For this review, use the dimensioned drawing (mm, ordinates from the lowest corner) and the shaded views. A direction names the side the tool comes from. Give positions to 0.01 mm unless a question says otherwise; leave off trailing zeros. Order: outer loops, then holes, each group sorted by start corner. A loop starts at its lowest first (then second) coordinate and runs counter-clockwise, first axis right, second up. Notation, with made-up numbers: (71, 89) - (117, 89) arc R30 ccw to (117, 121) - close; hole circle Ø9 at (38.25, 44.25). An arc over 180 degrees is marked (long way). Answer as CSV lines item,"result". Start each with the question number.
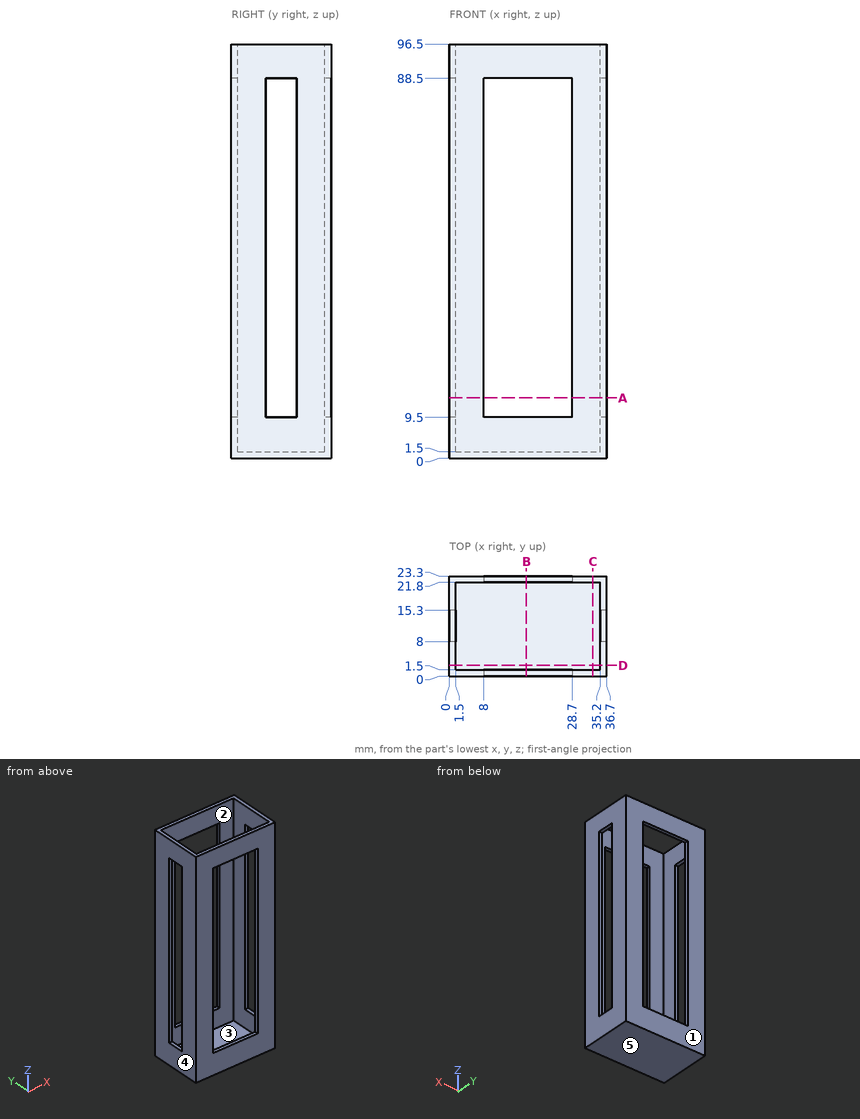
Item 1: Machinability: for the marked faces 1 and 2, which of the approach directions +Z, -Z, +X, -X, +Y, -Y give a long, thin tool a straight path to every point of the face, cutting with its end or side? Answer none if there is none.
Item 2: Take a section at B-B on x = 18. Write out the cut boundary in (y, z).
Item 3: For line 1 along X through (y, z) = (17, 81.5); line 2 along Y through (x, z) = (4, 33.5); line 3 along X through (y, z) = (1.25, 12), list the stretches that pass through material, from the lowest coordinate up.
Item 4: Clearance check with a flat-ended pin moving along its axis: pin 1 (3 mm diameter, centred on x = 19, y = 6.5, fed in from +Z). State where the tip first meets the part, or that it passes through.
Item 5: Take a section at D-D on y = 2.5. Write out the cut boundary in (x, z), and give its area (3 significant figures).
Item 6: Take a section at A-A on z = 14. Write out the cut boundary in (x, y).
Item 7: Mouldability with a two-part tool opening along X and no side actions: class the marked faces 3, 4 and 5 as released by +X, released by -X, zero draft, split by the parting line, or undercut.
Item 8: Take a section at C-C on x = 33.5. Write out the cut boundary in (y, z), and give its area (3 significant figures).
Data:
1,face 1,"+Z, -Z, +X, -X, +Y"
1,face 2,"+Z"
2,outline,"(0, 0) - (23.3, 0) - (23.3, 9.5) - (21.8, 9.5) - (21.8, 1.5) - (1.5, 1.5) - (1.5, 9.5) - (0, 9.5) - close; (0, 88.5) - (1.5, 88.5) - (1.5, 96.5) - (0, 96.5) - close; (21.8, 88.5) - (23.3, 88.5) - (23.3, 96.5) - (21.8, 96.5) - close"
3,line 1,"x = 0 to 1.5, 35.2 to 36.7"
3,line 2,"y = 0 to 1.5, 21.8 to 23.3"
3,line 3,"x = 0 to 8, 28.7 to 36.7"
4,pin 1,"stops at z = 1.5"
5,outline,"(0, 0) - (36.7, 0) - (36.7, 96.5) - (35.2, 96.5) - (35.2, 1.5) - (1.5, 1.5) - (1.5, 96.5) - (0, 96.5) - close"
5,area,"340 mm^2"
6,outline,"(0, 0) - (8, 0) - (8, 1.5) - (1.5, 1.5) - (1.5, 8) - (0, 8) - close; (0, 15.3) - (1.5, 15.3) - (1.5, 21.8) - (8, 21.8) - (8, 23.3) - (0, 23.3) - close; (28.7, 0) - (36.7, 0) - (36.7, 8) - (35.2, 8) - (35.2, 1.5) - (28.7, 1.5) - close; (28.7, 21.8) - (35.2, 21.8) - (35.2, 15.3) - (36.7, 15.3) - (36.7, 23.3) - (28.7, 23.3) - close"
7,face 3,"undercut"
7,face 4,"released by -X"
7,face 5,"zero draft"
8,outline,"(0, 0) - (23.3, 0) - (23.3, 96.5) - (21.8, 96.5) - (21.8, 1.5) - (1.5, 1.5) - (1.5, 96.5) - (0, 96.5) - close"
8,area,"320 mm^2"
